Design review of the part built by this model. Coordinates are the model's own, in mm. A direction names the side the tool comes from. Give positions to 0.01 mm unless a question says otherwise; leave off trailing zeros. Loops run counter-clockwise (first coordinate to the right, second up) from the corner with the lowest first, then second, coordinate; pieces in that order, holes last. Notation, with made-up numbers: M 25,77 L 69,77 A8 cw 69,86 Z; hole C 53,19 d5. An arc over 180 degrees is marked long. Use a Markdown table: item, result. Add a question column.
(1) Insertion check: pin 1 Ø1.5 at (x, y) = (1.5, 1.5) entering from +Z; pin 2 Ø3 at (x, z) = (50.5, -15) entering from -Y. Each pin has a flat end and moves straight along its axis. Give the tip position at first contact, or say it passes through.
(2) Add section A-A, the plane x = 4. Give the boundary of the cut face in (y, z), then the cut area to 3 significant figures.
(3) For faces 4 (the face through (0, 2, 30)), 5 (the face through (-59, 2, -43)), 6 (the face through (34, 1, 45)), list the 3-axis set-ups (+Z, -Z, +X, -X, +Y, -Y) from which the entire face can be reached by the end or side of a thin tool; tool diameter is ignored.
(4) Add section B-B, the plane z = 33. Give the boundary of the cut face in (x, y).
(5) Add section C-C, the plane y = 1.75. State how many separate pieces and enclosed holes the cut face has, then the cut area to 3 significant figures.
(6) Draft analysis for pull direction Z (two halves, no side actions). For faces 1 (the face through (-59, 2, 43)), 2 (the face through (60, 1, 1)), 3 (the face through (-6.597, 1.521, 61.904)), state which applies: pulls with the +Z half, pulls with the -Z half, needs draft (parallel to the pull), parting line crosses it, or undercut.
(7) Add section D-D, the plane z = -15. Give the boundary of the cut face in (x, y).
(8) For probe 1 along Z at (x, y) = (-22, 1); probe 2 along X at (y, z) = (1, -15); probe 3 along X at (y, z) = (0.7, 16), list the stretches that pass through material, from the lowest coordinate up.
```python
from build123d import *

# Parameters (mm, degrees)
SKETCH1_W           = 120
SKETCH1_H           = 90
BOSS_EXTRUDE1_DEPTH = 3
FILLET_1_R          = 5
CUT_EXTRUDE_1_DEPTH = 76.059976019
EXTRUDE_1_DEPTH     = 3
SKETCH_3_R          = 1.55
SKETCH_3_R_2        = 1.75
CUT_EXTRUDE_2_DEPTH = 103.055132159
FILLET_2_R          = 5


with BuildPart() as part:
    # Sketch1 → Boss-Extrude1 (new body)
    with BuildSketch(Plane(origin=(0, 0, 0), x_dir=(1, 0, 0), z_dir=(0, 1, 0))):
        Rectangle(SKETCH1_W, SKETCH1_H)
    extrude(amount=BOSS_EXTRUDE1_DEPTH)

    # 圆角1
    fillet_1_edges = [part.edges().sort_by_distance(p)[0] for p in [
        (60, 1.5, 45),
        (-60, 1.5, 45),
        (-60, 1.5, -45),
        (60, 1.5, -45),
    ]]
    fillet(fillet_1_edges, radius=FILLET_1_R)

    # 草图1 → 切除-拉伸1 (cut, through all)
    with BuildSketch(Plane(origin=(0, 3, 0), x_dir=(1, 0, 0), z_dir=(0, 1, 0))):
        with BuildLine():
            Line((-22.5, 36), (22.5, 36))
            ThreePointArc((22.5, 36), (25.5, 33), (22.5, 30))
            Line((22.5, 30), (-22.5, 30))
            ThreePointArc((-22.5, 30), (-25.5, 33), (-22.5, 36))
        make_face()
        with BuildLine():
            Line((-22.5, -30), (22.5, -30))
            ThreePointArc((22.5, -30), (25.5, -33), (22.5, -36))
            Line((22.5, -36), (-22.5, -36))
            ThreePointArc((-22.5, -36), (-25.5, -33), (-22.5, -30))
        make_face()
    extrude(amount=-CUT_EXTRUDE_1_DEPTH, mode=Mode.SUBTRACT)

    # 草图2 → 凸台-拉伸1 (add)
    with BuildSketch(Plane(origin=(0, 3, 0), x_dir=(1, 0, 0), z_dir=(0, 1, 0))):
        with BuildLine():
            Line((-10, -45), (10, -45))
            ThreePointArc((10, -45), (6.18491446, -59.768491446), (7, -75))
            ThreePointArc((7, -75), (-0.5, -82.5), (-8, -75))
            ThreePointArc((-8, -75), (-6.691600161, -59.846106677), (-10, -45))
        make_face()
    extrude(amount=-EXTRUDE_1_DEPTH)

    # 草图3 → 切除-拉伸2 (cut, through all)
    with BuildSketch(Plane(origin=(0, 3, 0), x_dir=(1, 0, 0), z_dir=(0, 1, 0))):
        with Locations(Location((42.5, -40, 0), (0, 0, 270))):
            Circle(SKETCH_3_R)
        with Locations(Location((42.5, 40, 0), (0, 0, 270))):
            Circle(SKETCH_3_R)
        with Locations(Location((-42.5, -40, 0), (0, 0, 270))):
            Circle(SKETCH_3_R)
        with Locations(Location((-42.5, 40, 0), (0, 0, 270))):
            Circle(SKETCH_3_R)
        with Locations(Location((-50.5, -15, 0), (0, 0, 270))):
            Circle(SKETCH_3_R_2)
        with Locations(Location((-26.5, -15, 0), (0, 0, 270))):
            Circle(SKETCH_3_R_2)
        with Locations(Location((-26.5, 15, 0), (0, 0, 270))):
            Circle(SKETCH_3_R_2)
        with Locations(Location((-50.5, 15, 0), (0, 0, 270))):
            Circle(SKETCH_3_R_2)
        with Locations(Location((50.5, -15, 0), (0, 0, 270))):
            Circle(SKETCH_3_R_2)
        with Locations(Location((50.5, 15, 0), (0, 0, 270))):
            Circle(SKETCH_3_R_2)
        with Locations(Location((26.5, -15, 0), (0, 0, 270))):
            Circle(SKETCH_3_R_2)
        with Locations(Location((26.5, 15, 0), (0, 0, 270))):
            Circle(SKETCH_3_R_2)
    extrude(amount=-CUT_EXTRUDE_2_DEPTH, mode=Mode.SUBTRACT)

    # 圆角2
    fillet_2_edges = [part.edges().sort_by_distance(p)[0] for p in [
        (10, 1.5, 45),
        (-10, 1.5, 45),
    ]]
    fillet(fillet_2_edges, radius=FILLET_2_R)


solid = part.part
```
Established:
| question | item | result |
|---|---|---|
| 1 | pin 1 | z = 82.4 |
| 1 | pin 2 | through |
| 2 | outline | M 0,-45 L 3,-45 L 3,-36 L 0,-36 Z; M 0,-30 L 3,-30 L 3,30 L 0,30 Z; M 0,36 L 3,36 L 3,81 L 0,81 Z |
| 2 | area | 342 mm^2 |
| 3 | face 4 | +Y, -Y |
| 3 | face 5 | -Z, -X, +Y, -Y |
| 3 | face 6 | +Z, +X, +Y, -Y |
| 4 | outline | M -60,0 L -25.5,0 L -25.5,3 L -60,3 Z; M 25.5,0 L 60,0 L 60,3 L 25.5,3 Z |
| 5 | separate pieces | 1 |
| 5 | enclosed holes | 14 |
| 5 | area | 10,600 mm^2 |
| 6 | face 1 | pulls with the +Z half |
| 6 | face 2 | needs draft |
| 6 | face 3 | undercut |
| 7 | outline | M -60,0 L -52.25,0 L -52.25,3 L -60,3 Z; M -48.75,0 L -28.25,0 L -28.25,3 L -48.75,3 Z; M -24.75,0 L 24.75,0 L 24.75,3 L -24.75,3 Z; M 28.25,0 L 48.75,0 L 48.75,3 L 28.25,3 Z; M 52.25,0 L 60,0 L 60,3 L 52.25,3 Z |
| 8 | probe 1 | -45 to -36, -30 to 30, 36 to 45 |
| 8 | probe 2 | -60 to -52.25, -48.75 to -28.25, -24.75 to 24.75, 28.25 to 48.75, 52.25 to 60 |
| 8 | probe 3 | -60 to -51.94, -49.06 to -27.94, -25.06 to 25.06, 27.94 to 49.06, 51.94 to 60 |
